Can you work these out from the drawing? Everything is in mm from the part's minimum corner. A direction names the side the tool comes from. Coordinates: 2 decimals unless noted, no trailing zeros. Loops run counter-clockwise (first coordinate to the right, second up) from the corner with the lowest first, then second, coordinate; pieces in that order, holes last.
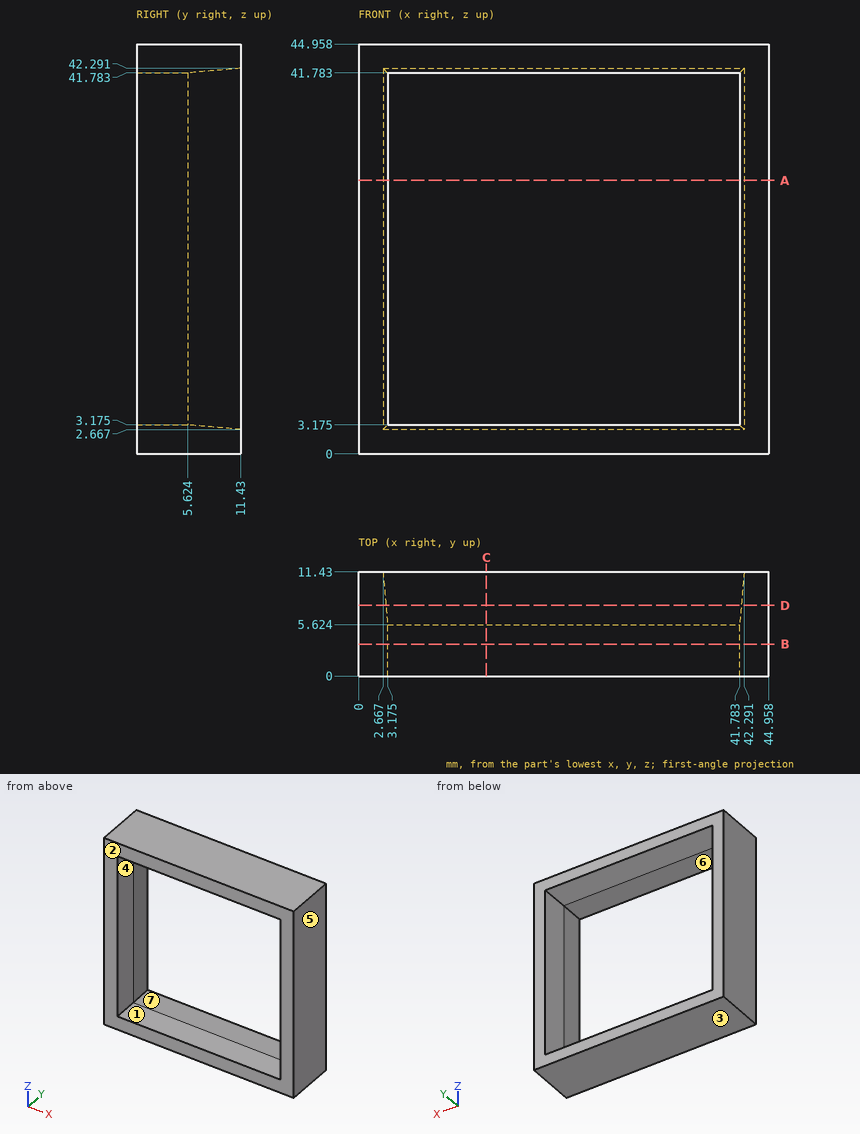
Item 1: On a 3-axis mill with a long thin cutter (end or side, diameter ignored), from which of +Z, -Z, +X, -X, +Y, -Y can I reach the whole of each face in a straight line? I mean the marked faces 5, 6 and 7. Say none if no direction works.
Results are:
face 5: +Z, -Z, +X, +Y, -Y
face 6: +Y, -Y
face 7: +Y
Item 2: I'm going to push flat-ended pins straight in: P1, Ø4.5, axis at x = 19.5, y = 1.5, coming from the -Z side; P2, Ø3, axis at x = 40, z = 21, coming from the -Y side. Where does each tip first touch, or does it pass through?
Results are:
P1: stops at z = 0
P2: passes through
Item 3: Suppose I cut it at B-B, the plane y = 3.5. Please give me the cut outline in (x, z) (1 decimal).
Results are:
outline: (0, 0) - (45, 0) - (45, 45) - (0, 45) - close; hole (3.2, 3.2) - (41.8, 3.2) - (41.8, 41.8) - (3.2, 41.8) - close
Item 4: I need wall thicknesses on line 1 along X through (y, z) = (1, 6) (1 decimal); line 2 along X through (y, z) = (7.75, 19.5). Which ranges of each line are inside material? Lowest first, please.
Results are:
line 1: x = 0 to 3.2, 41.8 to 45
line 2: x = 0 to 2.99, 41.97 to 44.96
Item 5: Suppose I cut it at D-D, the plane y = 7.75. Please give me the cut outline in (x, z).
Results are:
outline: (0, 0) - (44.96, 0) - (44.96, 44.96) - (0, 44.96) - close; hole (2.99, 2.99) - (41.97, 2.99) - (41.97, 41.97) - (2.99, 41.97) - close
Item 6: We'd pull the mould along Z, two halves only. Please class the marked faces 1, 2, 3 and 4: +Z half, -Z half, draft (parallel to the pull), parting line (faces both ways), or undercut.
Results are:
face 1: undercut
face 2: draft
face 3: -Z half
face 4: undercut
Item 7: Suppose I cut it at C-C, the plane x = 14. Please give me the cut outline in (y, z) (1 decimal).
Results are:
outline: (0, 0) - (11.4, 0) - (11.4, 2.7) - (5.6, 3.2) - (0, 3.2) - close; (0, 41.8) - (5.6, 41.8) - (11.4, 42.3) - (11.4, 45) - (0, 45) - close
Item 8: Suppose I cut it at A-A, the plane z = 30. Please give me the cut outline in (x, y) (1 decimal).
Results are:
outline: (0, 0) - (3.2, 0) - (3.2, 5.6) - (2.7, 11.4) - (0, 11.4) - close; (41.8, 0) - (45, 0) - (45, 11.4) - (42.3, 11.4) - (41.8, 5.6) - close
